Design review of the part built by this model. Coordinates are the model's own, in mm. A direction names the side the tool comes from. Round coordinates to 2 decimals unless told otherwise and drop trailing zeros. Order: outer loops, then holes, each group sorted by start corner. A loop starts at its lowest first (then second) coordinate and runs counter-clockwise, first axis right, second up. Notation, with made-up numbers: M 62,4 L 108,4 A24 cw 108,40 Z; hole C 89.25,-6.5 d5. An arc over 180 degrees is marked long. Use a Markdown table: item, result. Add a question column.
(1) Take a section at C-C (z = 9.25). Write out the cut boundary in (x, y).
(2) For pin 1 (5.5 mm diameter, centred on x = -1, z = 5.5, fed in from +Y); pin 2 (2 mm diameter, centred on x = -1, y = 5, fed in from +Z), all flat-tipped, find the tip position at first contact; note any pin that passes through.
(3) Take a section at B-B (y = 4). Write out the cut boundary in (x, z).
(4) Machinability: for faces 5 (the face through (0, 6, 0)), 6 (the face through (-9.1, 7.14, -0.99)), which of the approach directions +Z, -Z, +X, -X, +Y, -Y give a long, thin tool a straight path to every point of the face, cutting with its end or side? Answer none if there is none.
(5) Take a section at A-A (x = 6). Write out the cut boundary in (y, z), then the cut area to 3 significant figures.
(6) Take a section at D-D (x = 3.5). Write out the cut boundary in (y, z), then the cut area to 3 significant figures.
(7) To check wall thickness, follow probe 1 along X at (y, z) = (-1.4, 9); probe 2 along Y at (x, z) = (-3, 7.75); probe 3 along Y at (x, z) = (0, -1). State the ranges of each line that lie inside material, in increasing order. Write a range as from..to.
(8) The part is to be moulded in two halves that separate along Z. For faces 1 (the face through (0, -2, 6)), 2 (the face through (-5.93, -0.99, 7.5)), 3 (the face through (0, 6, -2)), 4 (the face through (0, -1, 12)), say which applies: released by +Z, released by -Z, zero draft, split by the parting line, or undercut.
```python
from build123d import *

# Parameters (mm, degrees)
BASE_FLANGE1_DEPTH = 10
FILLET1_R          = 3
SKETCH6_R          = 1.5
CUT_EXTRUDE1_DEPTH = 10
SKETCH7_R          = 1.5
CUT_EXTRUDE2_DEPTH = 10


# Sheet-metal steps are written as plain solids
with BuildPart() as part:
    # Sketch1 → Base-Flange1 (new, symmetric)
    with BuildSketch(Plane(origin=(0, 0, 0), x_dir=(0, 0, -1), z_dir=(1, 0, 0))):
        with BuildLine():
            Line((0, 8), (0, 0.7366))
            ThreePointArc((0, 0.7366), (-0.215745145, 0.215745145), (-0.7366, 0))
            Line((-0.7366, 0), (-12, 0))
            Line((-12, 0), (-12, -2))
            Line((-12, -2), (-0.7366, -2))
            ThreePointArc((-0.7366, -2), (1.198468417, -1.198468417), (2, 0.7366))
            Line((2, 0.7366), (2, 8))
            Line((2, 8), (0, 8))
        make_face()
    extrude(amount=BASE_FLANGE1_DEPTH, both=True)

    # Fillet1
    fillet1_edges = [part.edges().sort_by_distance(p)[0] for p in [
        (10, 8, -1),
        (10, -1, 12),
        (-10, 8, -1),
        (-10, -1, 12),
    ]]
    fillet(fillet1_edges, radius=FILLET1_R)

    # Sketch6 → Cut-Extrude1 (cut)
    with BuildSketch(Plane(origin=(0, 0, 0), x_dir=(1, 0, 0), z_dir=(0, 1, 0))):
        with Locations(Location((6, -9, 0), (0, 0, 270))):
            Circle(SKETCH6_R)
        with Locations(Location((-6, -9, 0), (0, 0, 270))):
            Circle(SKETCH6_R)
    extrude(amount=-CUT_EXTRUDE1_DEPTH, mode=Mode.SUBTRACT)

    # Sketch7 → Cut-Extrude2 (cut)
    with BuildSketch(Plane.XY):
        with Locations((0, 4)):
            Circle(SKETCH7_R)
    extrude(amount=-CUT_EXTRUDE2_DEPTH, mode=Mode.SUBTRACT)


solid = part.part
```
Verdict:
| question | item | result |
|---|---|---|
| 1 | outline | M -9.99,-2 L -7.48,-2 L -7.48,0 L -9.99,0 Z; M -4.52,-2 L 4.52,-2 L 4.52,0 L -4.52,0 Z; M 7.48,-2 L 9.99,-2 L 9.99,0 L 7.48,0 Z |
| 2 | pin 1 | stops at y = 0 |
| 2 | pin 2 | stops at z = 0 |
| 3 | outline | M -10,-2 L -1.5,-2 L -1.5,0 L -10,0 Z; M 1.5,-2 L 10,-2 L 10,0 L 1.5,0 Z |
| 4 | face 5 | +Z, +X, -X, +Y |
| 4 | face 6 | +Z, -Z, -X, +Y |
| 5 | outline | M -2,0.74 A2.74 ccw 0.74,-2 L 8,-2 L 8,0 L 0.74,0 A0.74 cw 0,0.74 L 0,7.5 L -2,7.5 Z; M -2,10.5 L 0,10.5 L 0,12 L -2,12 Z |
| 5 | area | 36.5 mm^2 |
| 6 | outline | M -2,0.74 A2.74 ccw 0.74,-2 L 8,-2 L 8,0 L 0.74,0 A0.74 cw 0,0.74 L 0,12 L -2,12 Z |
| 6 | area | 42.5 mm^2 |
| 7 | probe 1 | x = -10..-7.5, -4.5..4.5, 7.5..10 |
| 7 | probe 2 | y = -2..0 |
| 7 | probe 3 | y = -1.38..2.5, 5.5..8 |
| 8 | face 1 | zero draft |
| 8 | face 2 | undercut |
| 8 | face 3 | released by -Z |
| 8 | face 4 | released by +Z |
